from build123d import *

# Parameters (mm, degrees)
F1_DEPTH = 101.6


with BuildPart() as f1:
    # F0 (on Top) → F1 (new body)
    with BuildSketch(Plane.XY):
        with BuildLine():
            ThreePointArc((27.543169, 0), (-9.426531, 14.088715), (-46.396231, 0))
            Line((-46.396231, 0), (27.543169, 0))
        make_face()
        with BuildLine():
            Line((27.543169, 0), (-46.396231, 0))
            Line((-46.396231, 0), (-103.270147, -50.712894))
            Line((-103.270147, -50.712894), (-89.526953, -66.125726))
            Line((-89.526953, -66.125726), (-32.653037, -15.412831))
            ThreePointArc((-32.653037, -15.412831), (-9.426531, -6.561485), (13.799974, -15.412831))
            Line((13.799974, -15.412831), (70.673891, -66.125726))
            Line((70.673891, -66.125726), (84.417085, -50.712894))
            Line((84.417085, -50.712894), (27.543169, 0))
        make_face()
    extrude(amount=F1_DEPTH)


solid = f1.part
Could you check a few things on this model? Use its own coordinates, in mm. A direction names the side the tool comes from. Round coordinates to 2 decimals unless told otherwise and drop trailing zeros. Write each loop counter-clockwise with the first axis right and the second up, starting at its lowest first coordinate (ties: lowest second). Pieces come first, ordered by that corner, then holes. Notation, with made-up numbers: (79, -16.5) -> (97, -16.5) arc R17 cw to (97, -9.5) -> close; hole circle Ø3 at (75, 89). An arc over 180 degrees is marked (long way). Use a Markdown table: item, result.
1. Please list where these lines run through material, in increasing order: probe 1 along X at (y, z) = (-60, 74.5); probe 2 along X at (y, z) = (-48, 60); probe 3 along Y at (x, z) = (-81.5, 45).
Answer key:
| item | result |
|---|---|
| probe 1 | x = -94.99 to -82.66, 63.8 to 76.14 |
| probe 2 | x = -100.23 to -69.2, 50.35 to 81.37 |
| probe 3 | y = -58.97 to -31.3 |
2. If we section it at C-C (y = -59.5): List the corners of the cut face in (x, z) for me.
Answer key:
| item | result |
|---|---|
| outline | (-95.43, 0) -> (-82.1, 0) -> (-82.1, 101.6) -> (-95.43, 101.6) -> close; (63.24, 0) -> (76.58, 0) -> (76.58, 101.6) -> (63.24, 101.6) -> close |
3. For pin 1 Ø1 at (y, z) = (-49, 67) entering from -X; pin 2 Ø5 at (x, z) = (-48.5, 26.5) entering from +Y; pin 3 Ø4 at (x, z) = (-82.5, 42) entering from -Y; pin 4 Ø10 at (x, y) = (46.5, -6) entering from -Z, each with a flat end and sliding along its axis, tell me the tip position at first contact or that it passes through.
Answer key:
| item | result |
|---|---|
| pin 1 | stops at x = -101.91 |
| pin 2 | stops at y = 0.35 |
| pin 3 | stops at y = -61.64 |
| pin 4 | passes through |
4. If we section it at D-D (x = -55): List the corners of the cut face in (y, z) for me.
Answer key:
| item | result |
|---|---|
| outline | (-35.34, 0) -> (-7.67, 0) -> (-7.67, 101.6) -> (-35.34, 101.6) -> close |
5. We'd pull the mould along X, two halves only. Please class faces 3 (the face through (41.839, -40.414, 50.089)), 4 (the face through (-74.435, -25.001, 50.089)), 5 (the face through (-3, -5, 101.6)), 6 (the face through (77.449, -58.527, 50.089)): +X half, -X half, draft (parallel to the pull), parting line (faces both ways), or undercut.
Answer key:
| item | result |
|---|---|
| face 3 | undercut |
| face 4 | -X half |
| face 5 | draft |
| face 6 | +X half |
6. If we section it at A-A (z = 90): List the corners of the cut face in (x, y) for me.
Answer key:
| item | result |
|---|---|
| outline | (-103.27, -50.71) -> (-89.53, -66.13) -> (-32.65, -15.41) arc R34.9 cw to (13.8, -15.41) -> (70.67, -66.13) -> (84.42, -50.71) -> (27.54, 0) arc R55.55 ccw to (-46.4, 0) -> close |
7. Which directions (+Z, -Z, +X, -X, +Y, -Y) give clear straight access to the entire face, cutting with the end or side of a thin tool? Please do faces 1 (the face through (-61.488, -41.124, 50.089)), 2 (the face through (-3, -5, 0)).
Answer key:
| item | result |
|---|---|
| face 1 | +Z, -Z, -Y |
| face 2 | -Z, +X, -X, +Y, -Y |
8. If we section it at B-B (y = -24): List the corners of the cut face in (x, z) for me, then the cut area to 4 significant figures.
Answer key:
| item | result |
|---|---|
| outline | (-73.31, 0) -> (-42.28, 0) -> (-42.28, 101.6) -> (-73.31, 101.6) -> close; (23.43, 0) -> (54.46, 0) -> (54.46, 101.6) -> (23.43, 101.6) -> close |
| area | 6,305 mm^2 |
